For this review, take the finished solid that the model builds, in its own axes (mm). A direction names the side the tool comes from. Give positions to 0.01 mm unless a question says otherwise; leave off trailing zeros. Order: outer loops, then holes, each group sorted by start corner. A loop starts at its lowest first (then second) coordinate and runs counter-clockwise, first axis right, second up.
Item 1: For probe 1 along X at (y, z) = (14, -9); probe 2 along Z at (x, y) = (23, 32.5); probe 3 along Z at (x, y) = (-25, 15), list the stretches that pass through material, from the lowest coordinate up.
Item 2: For P1, Ø10, axis at x = 23.5, z = -8.5, coming from the +Y side; P2, Ø4.5, axis at x = -23, z = 9, coming from the -Y side; P3, Ø10, axis at x = -25, z = -9, coming from the +Y side; P4, Ø4.5, axis at x = 25, z = 9, coming from the +Y side, all flat-tipped, find the tip position at first contact; note any pin that passes through.
Item 3: Consider section B-B (y = 19.5). Give the boundary of the cut face in (x, z).
Item 4: Consider section C-C (z = 9.75). Give the boundary of the cut face in (x, y), plus the area to 3 significant figures.
Item 5: Machinability: for faces 4 (the flat face through (29, 15, 0)), 5 (the cylindrical face through (18.504, 31.625, 8.802)), 6 (the flat face through (5.9, 30.2, 5)), which of the approach directions +Z, -Z, +X, -X, +Y, -Y give a long, thin tool a straight path to every point of the face, cutting with its end or side? Answer none if there is none.
Item 6: Consider section A-A (x = 0). Give the boundary of the cut face in (y, z).
Item 7: Consider section D-D (z = -1). Give the boundary of the cut face in (x, y).
Item 8: The part is to be moulded in two halves that separate along Y. For faces 1 (the cylindrical face through (18.504, 31.625, -9.198)), 2 (the cylindrical face through (-3.47, 3.88, 10.07)), 3 (the flat face through (23, 27, 12)), say which applies: released by +Y, released by -Y, zero draft, split by the parting line, or undercut.
```python
from build123d import *

# Parameters (mm, degrees)
SZKIC1_W                                             = 58
SZKIC1_H                                             = 30
DODANIE_WYCI_GNI_CIE1_DEPTH                          = 42
SZKIC3_R                                             = 12
WYTNIJ_WYCI_GNI_CIE2_DEPTH                           = 60.203040462
SZKIC4_R                                             = 16
WYTNIJ_WYCI_GNI_CIE3_DEPTH                           = 10
POG_BIENIE_WALCOWE_POD_M5_WKR_T_DO_CZ_CI_D           = 5.5
POG_BIENIE_WALCOWE_POD_M5_WKR_T_DO_CZ_CI_CBORE_D     = 9
POG_BIENIE_WALCOWE_POD_M5_WKR_T_DO_CZ_CI_CBORE_DEPTH = 15
WYTNIJ_WYCI_GNI_CIE4_DEPTH                           = 60.203040462


with BuildPart() as part:
    # Szkic1 → Dodanie-wyciągnięcie1 (new body)
    with BuildSketch(Plane(origin=(0, 0, 0), x_dir=(1, 0, 0), z_dir=(0, 1, 0))):
        Rectangle(SZKIC1_W, SZKIC1_H)
    extrude(amount=DODANIE_WYCI_GNI_CIE1_DEPTH)

    # Szkic3 → Wytnij-wyciągnięcie2 (cut, through all)
    with BuildSketch(Plane.XY.offset(15)):
        with Locations((0, 19.5)):
            Circle(SZKIC3_R)
    extrude(amount=-WYTNIJ_WYCI_GNI_CIE2_DEPTH, mode=Mode.SUBTRACT)

    # Szkic4 → Wytnij-wyciągnięcie3 (cut)
    with BuildSketch(Plane.XY.offset(15)):
        with Locations((0, 19.5)):
            Circle(SZKIC4_R)
    wytnij_wyci_gni_cie3 = extrude(amount=-WYTNIJ_WYCI_GNI_CIE3_DEPTH, mode=Mode.SUBTRACT)

    # Lustro1: Wytnij-wyciągnięcie3 across plane
    add(wytnij_wyci_gni_cie3.mirror(Plane.XY), mode=Mode.SUBTRACT)

    # Pogłębienie walcowe pod M5 Wkręt do części metalowych z łbem sześciokątnym1 (through all)
    with Locations(Plane(origin=(0, 42, 0), x_dir=(1, 0, 0), z_dir=(0, 1, 0))):
        with Locations((-23, -9), (-23, 9), (23, -9), (23, 9)):
            CounterBoreHole(POG_BIENIE_WALCOWE_POD_M5_WKR_T_DO_CZ_CI_D / 2, POG_BIENIE_WALCOWE_POD_M5_WKR_T_DO_CZ_CI_CBORE_D / 2, POG_BIENIE_WALCOWE_POD_M5_WKR_T_DO_CZ_CI_CBORE_DEPTH)

    # Szkic10 → Wytnij-wyciągnięcie4 (cut, through all)
    with BuildSketch(Plane(origin=(0, 0, -15), x_dir=(-1, 0, 0), z_dir=(0, 0, -1))):
        Polygon((-29, 31.199169847), (-13.574815946, 42), (-29, 42), align=None)
        Polygon((13.574815946, 42), (29, 31.199169847), (29, 42), align=None)
    extrude(amount=-WYTNIJ_WYCI_GNI_CIE4_DEPTH, mode=Mode.SUBTRACT)


solid = part.part
```
Resolved:
1. probe 1: x = -29 to -25.75, -20.25 to -15.02, 15.02 to 20.25, 25.75 to 29
1. probe 2: z = -15 to -13.5, -4.5 to 4.5, 13.5 to 15
1. probe 3: z = -15 to -10.89, -7.11 to 7.11, 10.89 to 15
2. P1: stops at y = 38.55
2. P2: passes through
2. P3: stops at y = 35.53
2. P4: stops at y = 27
3. outline: (-29, -15) - (-16, -15) - (-16, -5) - (-12, -5) - (-12, 5) - (-16, 5) - (-16, 15) - (-29, 15) - close; (12, -5) - (16, -5) - (16, -15) - (29, -15) - (29, 15) - (16, 15) - (16, 5) - (12, 5) - close; hole circle Ø5.5 at (-23, -9); hole circle Ø5.5 at (-23, 9); hole circle Ø5.5 at (23, -9); hole circle Ø5.5 at (23, 9)
4. outline: (-29, 0) - (-25.65, 0) - (-25.65, 27) - (-27.44, 27) - (-27.44, 32.29) - (-29, 31.2) - close; (-20.35, 0) - (20.35, 0) - (20.35, 27) - (18.56, 27) - (18.56, 38.51) - (13.57, 42) - (-13.57, 42) - (-18.56, 38.51) - (-18.56, 27) - (-20.35, 27) - close; (25.65, 0) - (29, 0) - (29, 31.2) - (27.44, 32.29) - (27.44, 27) - (25.65, 27) - close; hole circle Ø32 at (0, 19.5)
4. area: 1,030 mm2
5. face 4: +Z, -Z, +X, +Y, -Y
5. face 5: +Y
5. face 6: +Z
6. outline: (0, -15) - (3.5, -15) - (3.5, -5) - (7.5, -5) - (7.5, 5) - (3.5, 5) - (3.5, 15) - (0, 15) - close; (31.5, -5) - (35.5, -5) - (35.5, -15) - (42, -15) - (42, 15) - (35.5, 15) - (35.5, 5) - (31.5, 5) - close
7. outline: (-29, 0) - (29, 0) - (29, 31.2) - (13.57, 42) - (-13.57, 42) - (-29, 31.2) - close; hole circle Ø24 at (0, 19.5)
8. face 1: zero draft
8. face 2: undercut
8. face 3: released by +Y
